```python
from build123d import *

# Parameters (mm, degrees)
F2_R     = 20
F3_DEPTH = 43.901
F4_SIZE  = 1


with BuildPart() as f1:
    # F0 (on Front) → F1 (revolve)
    with BuildSketch(Plane.XZ):
        Polygon((33.9, 9.525), (43.9, 9.525), (43.9, 20), (11.9, 20), (11.9, 13.225), (0, 13.225), (0, 9.525), (11.2, 9.525), (11.2, 8), (33.9, 8), align=None)
    revolve(axis=Axis((21.95, 0, 0), (1, 0, 0)))

    # F2 (on face) → F3 (cut, through all)
    with BuildSketch(Plane.YZ.offset(43.9)):
        Circle(F2_R)
        Polygon((-9.624429, 16.67), (9.624429, 16.67), (19.248858, 0), (9.624429, -16.67), (-9.624429, -16.67), (-19.248858, 0), align=None, mode=Mode.SUBTRACT)
    extrude(amount=-F3_DEPTH, mode=Mode.SUBTRACT)

    # F4
    f4_edges = [f1.edges().sort_by_distance(p)[0] for p in [
        (0, 0, -13.225),
    ]]
    chamfer(f4_edges, length=F4_SIZE)


solid = f1.part
```
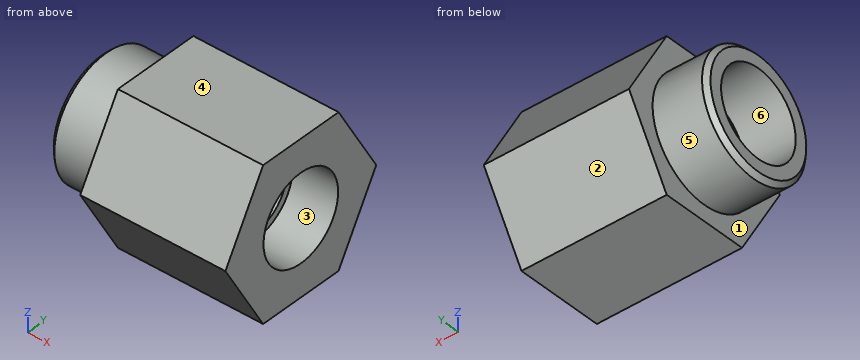
Input: part model. Units: mm. Frame: model coordinates. Face numbers are marked on the shaded views. A direction names the side the tool comes from. Round coordinates to 2 decimals unless told otherwise and drop trailing zeros. Loops run counter-clockwise (first coordinate to the right, second up) from the corner with the lowest first, then second, coordinate; pieces in that order, holes last. Notation, with made-up numbers: M 20,-15.75 L 75,-15.75 A18 cw 75,14.25 Z; hole C -21.75,83 d7. An arc over 180 degrees is marked long. Answer in a Markdown table with one row per item. Add a question column.
1. Contact query for flat-ended pins moving along their axis: pin 1 (3 mm diameter, centred on x = 26, z = 8, fed in from -Y); pin 2 (5 mm diameter, centred on x = 15, y = -12.5, fed in from +Z); pin 3 (9.5 mm diameter, centred on y = 4, z = -1, fed in from -X). Output: stop coordinate, or through.
2. Section B-B (y = 0). Output: boundary loops of the cut face in (x, z) (3 decimals), and give its area (3 significant figures).
3. Mould query, pull axis Y, two halves, no side actions, for the marked faces 4, 5 and 6. Classes: released by +Y, released by -Y, zero draft, split by the parting line, or undercut.
4. Ray query, probe 1 along Z at (x, y) = (19.5, 0); probe 2 along Z at (x, y) = (7, 0) (3 decimals); probe 3 along Y at (x, z) = (40, 0) (3 decimals). Return the intervals inside material, ascending.
5. Section C-C (y = -15.5). Output: boundary loops of the cut face in (x, z), and give its area (3 significant figures).
6. Set-up query: the marked faces 1, 2 and 3. Return all of +Z, -Z, +X, -X, +Y, -Y with unobstructed straight access to the full face (end or side cutting, diameter ignored); none if empty.
7. Section A-A (x = 25.5). Output: boundary loops of the cut face in (y, z).
Values follow:
| question | item | result |
|---|---|---|
| 1 | pin 1 | y = -15.5 |
| 1 | pin 2 | z = 16.02 |
| 1 | pin 3 | x = 11.2 |
| 2 | outline | M 0,-12.225 L 1,-13.225 L 11.9,-13.225 L 11.9,-16.67 L 43.9,-16.67 L 43.9,-9.525 L 33.9,-9.525 L 33.9,-8 L 11.2,-8 L 11.2,-9.525 L 0,-9.525 Z; M 0,9.525 L 11.2,9.525 L 11.2,8 L 33.9,8 L 33.9,9.525 L 43.9,9.525 L 43.9,16.67 L 11.9,16.67 L 11.9,13.225 L 1,13.225 L 0,12.225 Z |
| 2 | area | 614 mm^2 |
| 3 | face 4 | zero draft |
| 3 | face 5 | split by the parting line |
| 3 | face 6 | undercut |
| 4 | probe 1 | -16.67 to -8, 8 to 16.67 |
| 4 | probe 2 | -13.225 to -9.525, 9.525 to 13.225 |
| 4 | probe 3 | -19.249 to -9.525, 9.525 to 19.249 |
| 5 | outline | M 11.9,-6.49 L 43.9,-6.49 L 43.9,6.49 L 11.9,6.49 Z |
| 5 | area | 416 mm^2 |
| 6 | face 1 | -X |
| 6 | face 2 | -Z, +X, -X, +Y |
| 6 | face 3 | +X |
| 7 | outline | M -19.25,0 L -9.62,-16.67 L 9.62,-16.67 L 19.25,0 L 9.62,16.67 L -9.62,16.67 Z; hole C 0,0 d16 |
